Source: CAD feature listing. Evaluate the final solid. Frame: model axes, mm. Coordinates: 2 decimals unless noted, no trailing zeros. Loops run counter-clockwise (first coordinate to the right, second up) from the corner with the lowest first, then second, coordinate; pieces in that order, holes last.
Item 1: Section query A-A, the plane z = 1.3. Return the cut outline in (x, y) (1 decimal), then the cut area to 3 significant figures.
Item 2: Line query: probe 1 along Y at (x, z) = (0, 0.8); probe 2 along Y at (x, z) = (14.5, 1.2); probe 3 along X at (y, z) = (148, 2.65). Output: solid intervals per line, ascending.
Item 3: Section query C-C, the plane y = 137. Return the cut outline in (x, z) (3 decimals), then the cut area to 3 significant figures.
Item 4: Section query B-B, the plane x = -42.5. Return the cut outline in (y, z) (3 decimals), then the cut area to 3 significant figures.
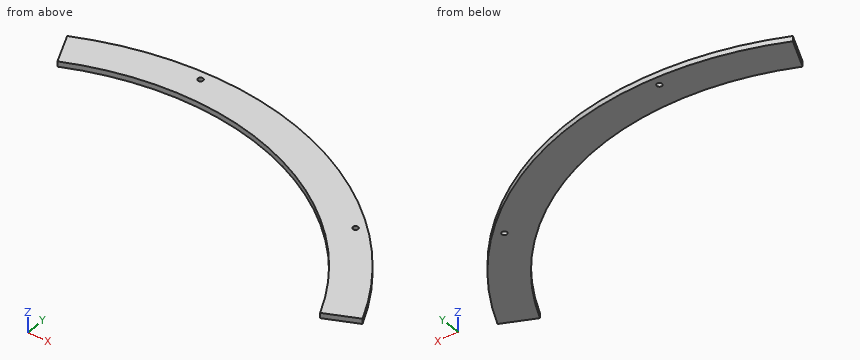
```python
from build123d import *

# Parameters (mm, degrees)
SKETCH2_R           = 190.5
SKETCH2_R_2         = 169.4688
BOSS_EXTRUDE2_DEPTH = 3.175
SKETCH6_R           = 1.5875
CUT_EXTRUDE1_DEPTH  = 270.426391849
SPLIT3_OUTLINE_R    = 1.5875
SPLIT3_DEPTH        = 3.175


# Read off the part's stored shape, not the designer's step: Split3
with BuildPart() as part:
    # Sketch2 → Boss-Extrude2 (new body)
    with BuildSketch(Plane.XY):
        Circle(SKETCH2_R)
        Circle(SKETCH2_R_2, mode=Mode.SUBTRACT)
    extrude(amount=BOSS_EXTRUDE2_DEPTH)

    # Sketch6 → Cut-Extrude1 (cut, through all)
    with BuildSketch(Plane.XY.offset(3.175)):
        with Locations((0, 184.785)):
            Circle(SKETCH6_R)
        with Locations((130.662726562, 130.662726562)):
            Circle(SKETCH6_R)
        with Locations((184.785, 0)):
            Circle(SKETCH6_R)
        with Locations((130.662726562, -130.662726562)):
            Circle(SKETCH6_R)
        with Locations((0, -184.785)):
            Circle(SKETCH6_R)
        with Locations((-130.662726562, -130.662726562)):
            Circle(SKETCH6_R)
        with Locations((-184.785, 0)):
            Circle(SKETCH6_R)
        with Locations((-130.662726562, 130.662726562)):
            Circle(SKETCH6_R)
    extrude(amount=-CUT_EXTRUDE1_DEPTH, mode=Mode.SUBTRACT)

    # Split3 outline → Split3 (cut)
    with BuildSketch(Plane.XY):
        with BuildLine():
            ThreePointArc((-72.901193866, 175.999050943), (-72.901193865, -175.999050944), (175.999050943, 72.901193866))
            Line((175.999050943, 72.901193866), (156.568755719, 64.852902063))
            ThreePointArc((156.568755719, 64.852902063), (-64.852902063, -156.568755719), (-64.852902063, 156.568755719))
            Line((-64.852902063, 156.568755719), (-72.901193866, 175.999050943))
        make_face()
        with Locations((-130.662726562, -130.662726562)):
            Circle(SPLIT3_OUTLINE_R, mode=Mode.SUBTRACT)
        with Locations((0, -184.785)):
            Circle(SPLIT3_OUTLINE_R, mode=Mode.SUBTRACT)
        with Locations((130.662726562, -130.662726562)):
            Circle(SPLIT3_OUTLINE_R, mode=Mode.SUBTRACT)
        with Locations((-184.785, 0)):
            Circle(SPLIT3_OUTLINE_R, mode=Mode.SUBTRACT)
        with Locations((-130.662726562, 130.662726562)):
            Circle(SPLIT3_OUTLINE_R, mode=Mode.SUBTRACT)
        with Locations((184.785, 0)):
            Circle(SPLIT3_OUTLINE_R, mode=Mode.SUBTRACT)
    extrude(amount=SPLIT3_DEPTH, mode=Mode.SUBTRACT)


solid = part.part
```
Verdict:
1. outline: (-72.9, 176) - (-64.9, 156.6) arc R169.5 cw to (156.6, 64.9) - (176, 72.9) arc R190.5 ccw to start; hole circle Ø3.2 at (0, 184.8); hole circle Ø3.2 at (130.7, 130.7)
1. area: 5,930 mm2
2. probe 1: y = 169.47 to 183.2, 186.37 to 190.5
2. probe 2: y = 168.85 to 189.95
2. probe 3: x = 82.56 to 119.94
3. outline: (99.753, 0) - (132.368, 0) - (132.368, 3.175) - (99.753, 3.175) - close
3. area: 104 mm2
4. outline: (164.053, 0) - (185.699, 0) - (185.699, 3.175) - (164.053, 3.175) - close
4. area: 68.7 mm2
